For this review, take the finished solid that the model builds, in its own axes (mm). A direction names the side the tool comes from. Give positions to 0.01 mm unless a question says otherwise; leave off trailing zeros. Write each loop counter-clockwise with the first axis right and the second up, starting at its lowest first coordinate (ties: lowest second). Pieces come first, ordered by that corner, then holes. Notation, with made-up numbers: (40, 3.25) -> (64, 3.25) arc R14 cw to (64, 25.25) -> close; hole circle Ø4 at (-9, 15). An arc over 180 degrees is marked (long way). Return JSON: item names as keys, results as strings.
Autodesk Inventor part; units mm, degrees
ref_plane "XY Plane" through (0, 0, 0) normal (0, 0, 1) x (1, 0, 0)
sketch "Block1" plane through (0, 0, 0) normal (0, 0, 1) x (1, 0, 0)
  line L0 (-0.685, 86) -> (2.315, 86)
  line L1 (-0.685, 86) -> (-0.685, 91)
  line L2 (2.315, 86) -> (1.4022, 87.742)
  line L3 (1.4022, 87.742) -> (1.4022, 89)
  line L4 (-0.5978, 91) -> (-0.685, 91)
  arc A0 (1.4022, 89) -> (-0.5978, 91) centre (-0.5978, 89) ccw
  point P0 (0.6511, 88.4856)
  dimension "d9" = 3
  dimension "d10" = 5
  dimension "d11" = 2
  dimension "d14" = 152.344
  dimension "d15" = 2.0871
sketch "Skizze1" plane through (0, 0, 0) normal (0, 0, 1) x (1, 0, 0)
  point P0 (0, 0)
sketch "Skizze2" plane through (0, 0, 0) normal (0, 0, 1) x (1, 0, 0)
  circle A0 centre (0, 0) radius 11.25
  dimension "d0" = 22.5
extrude "Extrusion1" add sketch "Skizze2" along normal blind 30
sketch "Skizze3" plane through (0, 0, 30) normal (0, 0, 1) x (1, 0, 0)
  circle A0 centre (0, 0) radius 11.25
  circle A1 centre (0, 0) radius 5
  dimension "d3" = 10
extrude "Extrusion2" add sketch "Skizze3" along normal blind 7 contours A1
sketch "Skizze4" plane through (0, 0, 37) normal (0, 0, 1) x (1, 0, 0)
  circle A0 centre (0, 0) radius 5
  circle A1 centre (0, 0) radius 2.5
  dimension "d6" = 5
extrude "Extrusion3" add sketch "Skizze4" along normal blind 6 contours A1
sketch "Skizze5" plane through (0, 0, 0) normal (1, 0, 0) x (0, 1, 0)
  line L0 (2.5, 43) -> (-2.5, 43)
  line L1 (-2.5, 43) -> (2.5, 43) construction
  line L2 (0, 43) -> (3, 43)
  line L3 (0, 43) -> (0, 48)
  line L4 (3, 43) -> (2.0871, 44.742)
  line L5 (2.0871, 44.742) -> (2.0871, 46)
  line L6 (0.0871, 48) -> (0, 48)
  arc A0 (2.0871, 46) -> (0.0871, 48) centre (0.0871, 46) ccw
  point P0 (0, 0)
sketch "Skizze6" plane through (0, 0, 0) normal (0, 0, -1) x (-1, 0, 0)
  circle A0 centre (0, 0) radius 11.25
  line L0 (7, 3.5) -> (7, -3.5)
  line L1 (7, -3.5) -> (8, -3.5)
  line L2 (7, 3.5) -> (8, 3.5)
  line L3 (8, -3.5) -> (8, 3.5)
  line L4 (0, 11.25) -> (0, -11.25) construction
  line L5 (-7, 3.5) -> (-7, -3.5)
  line L6 (-7, -3.5) -> (-8, -3.5)
  line L7 (-7, 3.5) -> (-8, 3.5)
  line L8 (-8, -3.5) -> (-8, 3.5)
  dimension "d19" = 7
  dimension "d20" = 1
  dimension "d21" = 7
  dimension "d23" = 3.5
extrude "Extrusion4" cut sketch "Skizze6" against normal blind 10
revolve "Umdrehung2" add sketch "Skizze5" angle 360 about axis through (0, 0, 43) along (0, 0, 1)
ref_plane "Arbeitsebene2" through (0, 5, 30) normal (0, 1, 0) x (-1, 0, 0)
ref_plane "Arbeitsebene1" through (0, 5, 30) normal (0, 1, 0) x (-1, 0, 0)
sketch "Skizze7" plane through (0, 5, 30) normal (0, 1, 0) x (-1, 0, 0)
  circle A0 centre (0, 3.4888) radius 2.5
  point P0 (0, -30)
  dimension "d27" = 5
extrude "Extrusion5" add sketch "Skizze7" along normal blind 15 and the other way blind 3
sketch "Skizze9" plane through (0, 0, 0) normal (1, 0, 0) x (0, 1, 0)
  point P0 (0, 0)
sketch "Skizze10" plane through (0, 0, 0) normal (1, 0, 0) x (0, 1, 0)
  point P0 (0, 0)
ref_plane "Arbeitsebene6" through (0, 0, 0) normal (1, 0, 0) x (0, 1, 0)
ref_plane "Arbeitsebene7" through (0, 20, 33.4888) normal (0, 1, 0) x (1, 0, 0)
sketch "Skizze11" plane through (0, 0, 0) normal (1, 0, 0) x (0, 1, 0)
  point P0 (0, 0)
sketch "Skizze12" plane through (0, 0, 0) normal (1, 0, 0) x (0, 1, 0)
  line L0 (0, 0) -> (0, 41.8024) construction
sketch "Skizze13" plane through (0, 0, 0) normal (1, 0, 0) x (0, 1, 0)
  line L0 (0, 43) -> (3, 43)
  line L1 (0, 43) -> (0, 48)
  line L2 (3, 43) -> (2.0871, 44.742)
  line L3 (2.0871, 44.742) -> (2.0871, 46)
  line L4 (0.0871, 48) -> (0, 48)
  arc A0 (2.0871, 46) -> (0.0871, 48) centre (0.0871, 46) ccw
  line L5 (19.9907, 33.5038) -> (19.9907, 30.5038)
  line L6 (19.9907, 33.5038) -> (24.9907, 33.5038)
  line L7 (19.9907, 30.5038) -> (21.7326, 31.4166)
  line L8 (21.7326, 31.4166) -> (22.9907, 31.4166)
  line L9 (24.9907, 33.4166) -> (24.9907, 33.5038)
  arc A1 (22.9907, 31.4166) -> (24.9907, 33.4166) centre (22.9907, 33.4166) ccw
  point P0 (0, 0)
revolve "Umdrehung3" add sketch "Skizze13" angle 360 about axis through (0, 19.9907, 33.5038) along (0, 1, 0) contours L6 L9 A1 L8 L7 L5
properties part number "Ventil_CPY"
1. Add section C-C, the plane y = 15. State the section outline as (x, z) points, plus the area to 3 significant figures.
Results found:
{"outline": "circle Ø5 at (0, 33.49)", "area": "19.6 mm²"}
2. To check wall thickness, follow probe 1 along Z at (x, y) = (-9.25, 3.5); probe 2 along Z at (x, y) = (0, 18); probe 3 along Z at (x, y) = (0.25, 10). State the ranges of each line that lie inside material, in increasing order.
Results found:
{"probe 1": "z = 10 to 30", "probe 2": "z = 30.99 to 35.99", "probe 3": "z = 10 to 30, 31 to 35.98"}
3. Add section A-A, the plane y = 7. State the section outline as (x, z) points.
Results found:
{"outline": "(-8.81, 10) -> (8.81, 10) -> (8.81, 30) -> (-8.81, 30) -> close; circle Ø5 at (0, 33.49)"}
4. Add section B-B, the plane z = 18. State the section outline as (x, y) points, plus the area to 3 significant figures.
Results found:
{"outline": "circle Ø22.5 at (0, 0)", "area": "398 mm²"}
5. For pin 1 (5 mm diameter, centred on y = 8, z = 13, fed in from -X); pin 2 (5.5 mm diameter, centred on y = -1.5, z = 3.5, fed in from -X); pin 3 (1 mm diameter, centred on x = -9, y = -4, fed in from -Z), all flat-tipped, find the tip position at first contact; note any pin that passes through.
Results found:
{"pin 1": "stops at x = -9.81", "pin 2": "stops at x = -8", "pin 3": "stops at z = 10"}
6. For faces 1 (the cylindrical face through (-0.09, 22.37, 35.59)), 2 (the flat face through (-2, -2, 43)), 3 (the flat face through (-7.5, -3.5, 4.9)), 4 (the flat face through (-7, 0, 5)), 5 (the flat face through (-8, 0, 5)), list the 3-axis set-ups (+Z, -Z, +X, -X, +Y, -Y) from which the entire face can be reached by the end or side of a thin tool; tool diameter is ignored.
Results found:
{"face 1": "+Y", "face 2": "none", "face 3": "-Z, +X, -X, -Y", "face 4": "-Z, +Y, -Y", "face 5": "-Z, -X, +Y, -Y"}
7. The part is to be moulded in two halves that separate along X. For faces 6 (the flat face through (7, 0, 5)), 7 (the cylindrical face through (-0.54, 2.44, 39.96)), 8 (the flat face through (7.5, 0, 0)), say which applies: +X half, -X half, draft (parallel to the pull), parting line (faces both ways), or undercut.
Results found:
{"face 6": "undercut", "face 7": "parting line", "face 8": "draft"}
